from build123d import *

# Parameters (mm, degrees)
CROQUIS1_W              = 200
CROQUIS1_H              = 45
SALIENTE_EXTRUIR1_DEPTH = 10
CORTAR_EXTRUIR1_REACH   = 104.987
CROQUIS2_R              = 3.25
CORTAR_EXTRUIR2_REACH   = 104.987
CROQUIS4_R              = 4.5
CORTAR_EXTRUIR3_REACH   = 104.987
CROQUIS6_R              = 1.75
CORTAR_EXTRUIR4_REACH   = 104.987
CROQUIS7_R              = 4
CROQUIS7_R_2            = 1.75
CROQUIS9_W              = 200
CROQUIS9_H              = 45
CROQUIS9_W_2            = 194
CROQUIS9_H_2            = 35
SALIENTE_EXTRUIR2_DEPTH = 5
REDONDEO1_R             = 10
REDONDEO2_R             = 10
CROQUIS10_R             = 1.75
CORTAR_EXTRUIR5_DEPTH   = 15
CROQUIS11_R             = 9.5
CROQUIS11_R_2           = 8
SALIENTE_EXTRUIR3_DEPTH = 4
REDONDEO3_R             = 3
CORTAR_EXTRUIR6_REACH   = 105.592
CROQUIS12_R             = 1.75
CROQUIS13_R             = 1.75
CORTAR_EXTRUIR7_DEPTH   = 10


with BuildPart() as part:
    # Croquis1 → Saliente-Extruir1 (new body)
    with BuildSketch(Plane(origin=(0, 0, 0), x_dir=(1, 0, 0), z_dir=(0, 1, 0))):
        Rectangle(CROQUIS1_W, CROQUIS1_H)
    extrude(amount=SALIENTE_EXTRUIR1_DEPTH)

    # Croquis2 → Cortar-Extruir1 (cut, up to next)
    with BuildSketch(Plane.XZ, mode=Mode.PRIVATE) as cortar_extruir1_sk1:
        with Locations(Location((-85, 0, 0), (0, 0, 270))):
            Circle(CROQUIS2_R)
    cortar_extruir1_tool1 = extrude(cortar_extruir1_sk1.sketch, amount=-CORTAR_EXTRUIR1_REACH, mode=Mode.PRIVATE) & part.part
    add(cortar_extruir1_tool1.solids().sort_by_distance((-85, 0, 0))[0], mode=Mode.SUBTRACT)

    # Croquis4 → Cortar-Extruir2 (cut, up to next)
    with BuildSketch(Plane(origin=(0, 10, 0), x_dir=(1, 0, 0), z_dir=(0, 1, 0)), mode=Mode.PRIVATE) as cortar_extruir2_sk1:
        with Locations(Location((76, 0, 0), (0, 0, 270))):
            Circle(CROQUIS4_R)
    cortar_extruir2_tool1 = extrude(cortar_extruir2_sk1.sketch, amount=-CORTAR_EXTRUIR2_REACH, mode=Mode.PRIVATE) & part.part
    add(cortar_extruir2_tool1.solids().sort_by_distance((76, 10, 0))[0], mode=Mode.SUBTRACT)

    # Croquis6 → Cortar-Extruir3 (cut, up to next)
    with BuildSketch(Plane.XZ, mode=Mode.PRIVATE) as cortar_extruir3_sk1:
        with Locations(Location((-77, 0, 0), (0, 0, 270))):
            Circle(CROQUIS6_R)
    cortar_extruir3_tool1 = extrude(cortar_extruir3_sk1.sketch, amount=-CORTAR_EXTRUIR3_REACH, mode=Mode.PRIVATE) & part.part
    # Croquis6 → Cortar-Extruir3 (cut, up to next)
    with BuildSketch(Plane.XZ, mode=Mode.PRIVATE) as cortar_extruir3_sk2:
        with Locations(Location((-93, 0, 0), (0, 0, 270))):
            Circle(CROQUIS6_R)
    cortar_extruir3_tool2 = extrude(cortar_extruir3_sk2.sketch, amount=-CORTAR_EXTRUIR3_REACH, mode=Mode.PRIVATE) & part.part
    # Croquis6 → Cortar-Extruir3 (cut, up to next)
    with BuildSketch(Plane.XZ, mode=Mode.PRIVATE) as cortar_extruir3_sk3:
        with Locations(Location((-85, 8, 0), (0, 0, 270))):
            Circle(CROQUIS6_R)
    cortar_extruir3_tool3 = extrude(cortar_extruir3_sk3.sketch, amount=-CORTAR_EXTRUIR3_REACH, mode=Mode.PRIVATE) & part.part
    # Croquis6 → Cortar-Extruir3 (cut, up to next)
    with BuildSketch(Plane.XZ, mode=Mode.PRIVATE) as cortar_extruir3_sk4:
        with Locations(Location((-85, -8, 0), (0, 0, 270))):
            Circle(CROQUIS6_R)
    cortar_extruir3_tool4 = extrude(cortar_extruir3_sk4.sketch, amount=-CORTAR_EXTRUIR3_REACH, mode=Mode.PRIVATE) & part.part
    add(cortar_extruir3_tool1.solids().sort_by_distance((-77, 0, 0))[0], mode=Mode.SUBTRACT)
    add(cortar_extruir3_tool2.solids().sort_by_distance((-93, 0, 0))[0], mode=Mode.SUBTRACT)
    add(cortar_extruir3_tool3.solids().sort_by_distance((-85, 0, 8))[0], mode=Mode.SUBTRACT)
    add(cortar_extruir3_tool4.solids().sort_by_distance((-85, 0, -8))[0], mode=Mode.SUBTRACT)

    # Croquis7 → Cortar-Extruir4 (cut, up to next)
    with BuildSketch(Plane.XZ, mode=Mode.PRIVATE) as cortar_extruir4_sk1:
        with Locations(Location((-58, 0, 0), (0, 0, 270))):
            Circle(CROQUIS7_R)
    cortar_extruir4_tool1 = extrude(cortar_extruir4_sk1.sketch, amount=-CORTAR_EXTRUIR4_REACH, mode=Mode.PRIVATE) & part.part
    # Croquis7 → Cortar-Extruir4 (cut, up to next)
    with BuildSketch(Plane.XZ, mode=Mode.PRIVATE) as cortar_extruir4_sk2:
        with Locations(Location((-58, 8.5, 0), (0, 0, 270))):
            Circle(CROQUIS7_R_2)
    cortar_extruir4_tool2 = extrude(cortar_extruir4_sk2.sketch, amount=-CORTAR_EXTRUIR4_REACH, mode=Mode.PRIVATE) & part.part
    # Croquis7 → Cortar-Extruir4 (cut, up to next)
    with BuildSketch(Plane.XZ, mode=Mode.PRIVATE) as cortar_extruir4_sk3:
        with Locations(Location((-58, -8.5, 0), (0, 0, 270))):
            Circle(CROQUIS7_R_2)
    cortar_extruir4_tool3 = extrude(cortar_extruir4_sk3.sketch, amount=-CORTAR_EXTRUIR4_REACH, mode=Mode.PRIVATE) & part.part
    add(cortar_extruir4_tool1.solids().sort_by_distance((-58, 0, 0))[0], mode=Mode.SUBTRACT)
    add(cortar_extruir4_tool2.solids().sort_by_distance((-58, 0, 8.5))[0], mode=Mode.SUBTRACT)
    add(cortar_extruir4_tool3.solids().sort_by_distance((-58, 0, -8.5))[0], mode=Mode.SUBTRACT)

    # Croquis9 → Saliente-Extruir2 (add)
    with BuildSketch(Plane.XZ):
        Rectangle(CROQUIS9_W, CROQUIS9_H)
        Rectangle(CROQUIS9_W_2, CROQUIS9_H_2, mode=Mode.SUBTRACT)
    extrude(amount=SALIENTE_EXTRUIR2_DEPTH)

    # Redondeo1
    redondeo1_edges = [part.edges().sort_by_distance(p)[0] for p in [
        (100, 2.5, 22.5),
        (-100, 2.5, 22.5),
        (-100, 2.5, -22.5),
        (100, 2.5, -22.5),
    ]]
    fillet(redondeo1_edges, radius=REDONDEO1_R)

    # Redondeo2
    redondeo2_edges = [part.edges().sort_by_distance(p)[0] for p in [
        (97, -2.5, 17.5),
        (-97, -2.5, 17.5),
        (-97, -2.5, -17.5),
        (97, -2.5, -17.5),
    ]]
    fillet(redondeo2_edges, radius=REDONDEO2_R)

    # Croquis10 → Cortar-Extruir5 (cut)
    with BuildSketch(Plane.XZ.offset(5)):
        with Locations(Location((88, 20, 0), (0, 0, 270))):
            Circle(CROQUIS10_R)
        with Locations(Location((62, 20, 0), (0, 0, 270))):
            Circle(CROQUIS10_R)
        with Locations(Location((62, -20, 0), (0, 0, 270))):
            Circle(CROQUIS10_R)
        with Locations(Location((88, -20, 0), (0, 0, 270))):
            Circle(CROQUIS10_R)
    extrude(amount=-CORTAR_EXTRUIR5_DEPTH, mode=Mode.SUBTRACT)

    # Croquis11 → Saliente-Extruir3 (add)
    with BuildSketch(Plane.XZ):
        with Locations(Location((76, 0, 0), (0, 0, 270))):
            Circle(CROQUIS11_R)
        with Locations(Location((76, 0, 0), (0, 0, 270))):
            Circle(CROQUIS11_R_2, mode=Mode.SUBTRACT)
    extrude(amount=SALIENTE_EXTRUIR3_DEPTH)

    # Redondeo3
    redondeo3_edges = [part.edges().sort_by_distance(p)[0] for p in [
        (76, 0, 9.5),
    ]]
    fillet(redondeo3_edges, radius=REDONDEO3_R)

    # Croquis12 → Cortar-Extruir6 (cut, up to next)
    with BuildSketch(Plane(origin=(0, 10, 0), x_dir=(1, 0, 0), z_dir=(0, 1, 0)), mode=Mode.PRIVATE) as cortar_extruir6_sk1:
        with Locations(Location((91, 0, 0), (0, 0, 270))):
            Circle(CROQUIS12_R)
    cortar_extruir6_tool1 = extrude(cortar_extruir6_sk1.sketch, amount=-CORTAR_EXTRUIR6_REACH, mode=Mode.PRIVATE) & part.part
    add(cortar_extruir6_tool1.solids().sort_by_distance((91, 10, 0))[0], mode=Mode.SUBTRACT)

    # Croquis13 → Cortar-Extruir7 (cut)
    with BuildSketch(Plane(origin=(0, 10, 0), x_dir=(1, 0, 0), z_dir=(0, 1, 0))):
        with Locations(Location((28.353351566, -12.5, 0), (0, 0, 270))):
            Circle(CROQUIS13_R)
        with Locations(Location((13.353351566, -12.5, 0), (0, 0, 270))):
            Circle(CROQUIS13_R)
        with Locations(Location((-1.646648434, -12.5, 0), (0, 0, 270))):
            Circle(CROQUIS13_R)
        with Locations(Location((-16.646648434, -12.5, 0), (0, 0, 270))):
            Circle(CROQUIS13_R)
        with Locations(Location((-31.646648434, -12.5, 0), (0, 0, 270))):
            Circle(CROQUIS13_R)
        with Locations(Location((-46.646648434, -12.5, 0), (0, 0, 270))):
            Circle(CROQUIS13_R)
    extrude(amount=-CORTAR_EXTRUIR7_DEPTH, mode=Mode.SUBTRACT)


solid = part.part
Geometry check sheet. Reference: the model listing, model coordinates, mm. A direction names the side the tool comes from. Round coordinates to 2 decimals unless told otherwise and drop trailing zeros. Order: outer loops, then holes, each group sorted by start corner. A loop starts at its lowest first (then second) coordinate and runs counter-clockwise, first axis right, second up. Notation, with made-up numbers: M 32.25,71.25 L 50.25,71.25 A17 cw 50.25,77.25 Z; hole C 58.5,57.25 d9. An arc over 180 degrees is marked long. Answer in a Markdown table with one row per item. Add a question column.
Item 1: Sectioned sample at A-A, the plane x = -85. Enter the section's corners in (y, z).
Item 2: Sectioned sample at B-B, the plane x = 76. Enter the section's corners in (y, z).
Item 3: Sectioned sample at C-C, the plane y = 7.25. State how many separate pieces and enclosed holes the cut face has, plus the area to 3 significant figures.
Item 4: Set-up check for faces 3 (the face through (60.29, 2.39, -19.62)), 4 (the face through (97, -2, 0)): record each of +Z, -Z, +X, -X, +Y, -Y from which the full face is reachable in a straight line by a thin tool's end or side.
Item 5: Draft check along Z on faces 1 (the face through (-1, 10, 0)), 2 (the face through (-86.71, 4.93, -7.62)). Enter one of: released by +Z, released by -Z, zero draft, split by the parting line, or undercut.
Item 6: Depth check by flat-ended pin: pin 1 Ø4 at (x, z) = (91, 0) entering from -Y; pin 2 Ø3 at (x, z) = (62, -20) entering from +Y. Enter the tip coordinate at first touch or a pass-through.
Item 7: Material ranges on L1, parallel to Z at x = 73.5, y = -2.5; L2, parallel to X at y = 3.75, z = 8; L3, parallel to X at y = 5.5, z = 20, recorded low to high. Write a range as [from, to].
Filled in:
| question | item | result |
|---|---|---|
| 1 | outline | M -5,-22.5 L 10,-22.5 L 10,-9.75 L 0,-9.75 L 0,-17.5 L -5,-17.5 Z; M -5,17.5 L 0,17.5 L 0,9.75 L 10,9.75 L 10,22.5 L -5,22.5 Z; M 0,-6.25 L 10,-6.25 L 10,-3.25 L 0,-3.25 Z; M 0,3.25 L 10,3.25 L 10,6.25 L 0,6.25 Z |
| 2 | outline | M -5,-22.5 L 10,-22.5 L 10,-4.5 L 0,-4.5 L 0,-8 L -4,-8 L -4,-9.5 L -3,-9.5 A3 cw 0,-12.5 L 0,-17.5 L -5,-17.5 Z; M -5,17.5 L 0,17.5 L 0,12.5 A3 cw -3,9.5 L -4,9.5 L -4,8 L 0,8 L 0,4.5 L 10,4.5 L 10,22.5 L -5,22.5 Z |
| 3 | separate pieces | 1 |
| 3 | enclosed holes | 20 |
| 3 | area | 8,600 mm² |
| 4 | face 3 | +Y, -Y |
| 4 | face 4 | -Y |
| 5 | face 1 | zero draft |
| 5 | face 2 | undercut |
| 6 | pin 1 | stops at y = 0 |
| 6 | pin 2 | passes through |
| 7 | L1 | z = [-22.5, -17.5], [-9.21, -7.6], [7.6, 9.21], [17.5, 22.5] |
| 7 | L2 | x = [-100, -86.75], [-83.25, -59.68], [-56.32, 100] |
| 7 | L3 | x = [-96.61, 60.25], [63.75, 86.25], [89.75, 96.61] |
